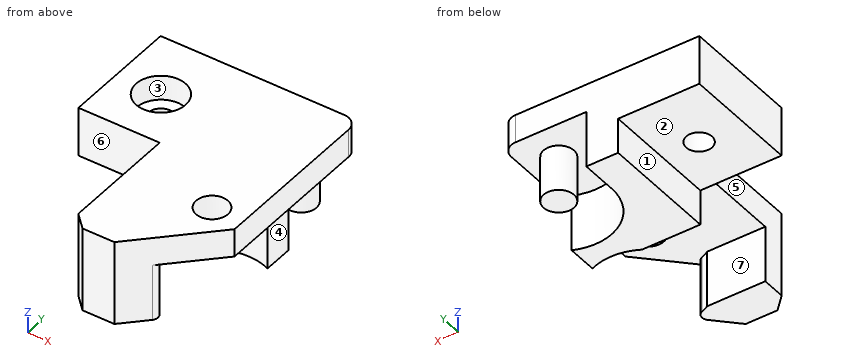
```python
from build123d import *

# Parameters (mm, degrees)
BOSS_EXTRUDE1_DEPTH                            = 4
SKETCH2_R                                      = 2.25
CUT_EXTRUDE1_DEPTH                             = 46
SKETCH2_3_R                                    = 2.15
BOSS_EXTRUDE2_DEPTH                            = 8
BOSS_EXTRUDE4_DEPTH                            = 8
SKETCH6_W                                      = 11.5
SKETCH6_H                                      = 18.413961031
CUT_EXTRUDE2_DEPTH                             = 47.400431032
SKETCH12_W                                     = 8
SKETCH12_H                                     = 13.1
CUT_EXTRUDE3_DEPTH                             = 40.286161686
CBORE_FOR_6_SOCKET_HEAD_CAP_SCREW1_D           = 3.6576
CBORE_FOR_6_SOCKET_HEAD_CAP_SCREW1_CBORE_D     = 7
CBORE_FOR_6_SOCKET_HEAD_CAP_SCREW1_CBORE_DEPTH = 3.5052
SKETCH13_W                                     = 11.5
SKETCH13_H                                     = 16.586038969
CUT_EXTRUDE4_DEPTH                             = 5
CHAMFER1_SIZE                                  = 2
CUT_EXTRUDE5_START                             = -1.5
SKETCH14_R                                     = 2.15
CUT_EXTRUDE5_DEPTH                             = 1.5


with BuildPart() as part:
    # Sketch1 → Boss-Extrude1 (new body)
    with BuildSketch(Plane.XY):
        with BuildLine():
            Line((18, 0), (28, 10))
            Line((28, 10), (28, 33))
            ThreePointArc((28, 33), (27.414213562, 34.414213562), (26, 35))
            Line((26, 35), (0, 35))
            Line((0, 35), (0, 0))
            Line((0, 0), (18, 0))
        make_face()
    extrude(amount=BOSS_EXTRUDE1_DEPTH)

    # Sketch2 → Cut-Extrude1 (cut, through all)
    with BuildSketch(Plane(origin=(0, 0, 0), x_dir=(-1, 0, 0), z_dir=(0, 0, -1))):
        with Locations((-23.5, 11.863961031)):
            Circle(SKETCH2_R)
    extrude(amount=-CUT_EXTRUDE1_DEPTH, mode=Mode.SUBTRACT)

    # Sketch2<3> → Boss-Extrude2 (add)
    with BuildSketch(Plane(origin=(0, 0, 0), x_dir=(-1, 0, 0), z_dir=(0, 0, -1))):
        with Locations(Location((-23.5, 29.863961031, 0), (0, 0, 180))):
            Circle(SKETCH2_3_R)
    extrude(amount=BOSS_EXTRUDE2_DEPTH)

    # Sketch2<5> → Boss-Extrude4 (add)
    with BuildSketch(Plane(origin=(0, 0, 0), x_dir=(-1, 0, 0), z_dir=(0, 0, -1))):
        with BuildLine():
            ThreePointArc((-26.5, 18.792344681), (-23.077745882, 19.402143932), (-19.745003329, 18.413961031))
            Line((-19.745003329, 18.413961031), (-15.95, 18.413961031))
            Line((-15.95, 18.413961031), (-15.95, 5.313961031))
            Line((-15.95, 5.313961031), (-19.725, 5.313961031))
            ThreePointArc((-19.725, 5.313961031), (-20.25595921, 5.035394245), (-20.807324798, 4.799782009))
            ThreePointArc((-20.807324798, 4.799782009), (-21.429052247, 4.074422526), (-21.15825613, 3.15825613))
            Line((-21.15825613, 3.15825613), (-18, 0))
            Line((-18, 0), (0, 0))
            Line((0, 0), (0, 35))
            Line((0, 35), (-16, 35))
            Line((-16, 35), (-16, 29.863961031))
            ThreePointArc((-16, 29.863961031), (-19.392080819, 23.589010832), (-26.5, 22.990097488))
            Line((-26.5, 22.990097488), (-26.5, 18.792344681))
        make_face()
    extrude(amount=BOSS_EXTRUDE4_DEPTH)

    # Sketch6 → Cut-Extrude2 (cut, through all)
    with BuildSketch(Plane(origin=(0, 0, -8), x_dir=(-1, 0, 0), z_dir=(0, 0, -1))):
        with Locations((-5.75, 9.206980515)):
            Rectangle(SKETCH6_W, SKETCH6_H)
    extrude(amount=-CUT_EXTRUDE2_DEPTH, mode=Mode.SUBTRACT)

    # Sketch12 → Cut-Extrude3 (cut, through all)
    with BuildSketch(Plane(origin=(15.95, 0, 0), x_dir=(0, 0, -1), z_dir=(1, 0, 0))):
        with Locations((4, 11.863961031)):
            Rectangle(SKETCH12_W, SKETCH12_H)
    extrude(amount=-CUT_EXTRUDE3_DEPTH, mode=Mode.SUBTRACT)

    # CBORE for #6 Socket Head Cap Screw1 (through all)
    with Locations(Plane.XY.offset(4)):
        with Locations((6.35, 26)):
            CounterBoreHole(CBORE_FOR_6_SOCKET_HEAD_CAP_SCREW1_D / 2, CBORE_FOR_6_SOCKET_HEAD_CAP_SCREW1_CBORE_D / 2, CBORE_FOR_6_SOCKET_HEAD_CAP_SCREW1_CBORE_DEPTH)

    # Sketch13 → Cut-Extrude4 (cut)
    with BuildSketch(Plane(origin=(0, 0, -8), x_dir=(-1, 0, 0), z_dir=(0, 0, -1))):
        with Locations((-5.75, 26.706980515)):
            Rectangle(SKETCH13_W, SKETCH13_H)
    extrude(amount=-CUT_EXTRUDE4_DEPTH, mode=Mode.SUBTRACT)

    # Chamfer1
    chamfer1_edges = [part.edges().sort_by_distance(p)[0] for p in [
        (11.5, 0, -2),
    ]]
    chamfer(chamfer1_edges, length=CHAMFER1_SIZE)

    # Sketch14 → Cut-Extrude5 (cut)
    with BuildSketch(Plane(origin=(0, 0, -8), x_dir=(-1, 0, 0), z_dir=(0, 0, -1)).offset(CUT_EXTRUDE5_START)):
        with Locations(Location((-23.5, 29.863961031, 0), (0, 0, 180))):
            Circle(SKETCH14_R)
    extrude(amount=CUT_EXTRUDE5_DEPTH, mode=Mode.SUBTRACT)


solid = part.part
```
Check sheet for the modelled part. Datum: model origin and axes. Units: mm. Face numbers are marked on the shaded views. A direction names the side the tool comes from. Round coordinates to 2 decimals unless told otherwise and drop trailing zeros. Order: outer loops, then holes, each group sorted by start corner. A loop starts at its lowest first (then second) coordinate and runs counter-clockwise, first axis right, second up. Notation, with made-up numbers: (44, 20.25) - (86, 20.25) arc R21 cw to (86, 30.25) - close; hole circle Ø10 at (9, -22). An arc over 180 degrees is marked (long way). Answer as CSV lines item,"result". Start each with the question number.
1) Scan lines: probe 1 along Y at (x, z) = (6.35, 2.05); probe 2 along Y at (x, z) = (6.35, -1.8); probe 3 along Z at (x, y) = (8, 24). Record each from-to range of solid material in increasing order.
2) Section check B-B (z = -1). Record the cut outline in (x, y) (3 decimals), then the cut area to 3 significant figures.
3) Tool access check on the marked faces 4, 5, 6 and 7. Record the directions out of +Z, -Z, +X, -X, +Y, -Y that give a thin tool (end or side, any length) a straight path to the whole face; none if there is none.
4) Draft check along X on the marked faces 1, 2 and 3. Enter one of: +X half, -X half, draft (parallel to the pull), parting line (faces both ways), or undercut.
5) Section check A-A (x = 6.35). Record the cut outline in (y, z).
6) Section check D-D (z = 1.25). Record the cut outline in (x, y).
7) Section check C-C (y = 26). Record the cut outline in (x, z).
8) Depth check by flat-ended pin: pin 1 (12 mm diameter, centred on x = 23.5, y = 13.5, fed in from -Z); pin 2 (2.5 mm diameter, centred on y = 30, z = -6.5, fed in from -X); pin 3 (6 mm diameter, centred on x = 7, z = -5, fed in from -Y); pin 4 (3.5 mm diameter, centred on x = 24, y = 29.5, fed in from -Z). Enter the tip coordinate at first touch or a pass-through.
Determined:
1,probe 1,"18.41 to 22.5, 29.5 to 35"
1,probe 2,"18.41 to 24.17, 27.83 to 35"
1,probe 3,"-3 to 0.49"
2,outline,"(0, 18.414) - (19.745, 18.414) arc R7.55 cw to (26.5, 18.792) - (26.5, 22.99) arc R7.5 cw to (16, 29.864) - (16, 35) - (0, 35) - close; (11.5, 2) - (13.5, 0) - (18, 0) - (21.158, 3.158) arc R1 ccw to (20.807, 4.8) arc R7.56 cw to (19.725, 5.314) - (11.5, 5.314) - close; circle Ø4.3 at (23.5, 29.864); hole circle Ø3.658 at (6.35, 26)"
2,area,"363 mm^2"
3,face 4,"-Z, +X, +Y, -Y"
3,face 5,"+Z, -Z, -X, -Y"
3,face 6,"-Z, -X"
3,face 7,"-Z, +X, -X"
4,face 1,"-X half"
4,face 2,"draft"
4,face 3,"undercut"
5,outline,"(18.41, -3) - (24.17, -3) - (24.17, 0.49) - (22.5, 0.49) - (22.5, 4) - (18.41, 4) - close; (27.83, -3) - (35, -3) - (35, 4) - (29.5, 4) - (29.5, 0.49) - (27.83, 0.49) - close"
6,outline,"(0, 18.41) - (11.5, 18.41) - (11.5, 2) - (13.5, 0) - (18, 0) - (28, 10) - (28, 33) arc R2 ccw to (26, 35) - (0, 35) - close; hole circle Ø7 at (6.35, 26); hole circle Ø4.5 at (23.5, 11.86)"
7,outline,"(0, -3) - (4.52, -3) - (4.52, 0.49) - (2.85, 0.49) - (2.85, 4) - (0, 4) - close; (8.18, -3) - (11.5, -3) - (11.5, -8) - (17.07, -8) - (17.07, 0) - (28, 0) - (28, 4) - (9.85, 4) - (9.85, 0.49) - (8.18, 0.49) - close"
8,pin 1,"z = -8"
8,pin 2,"x = 11.5"
8,pin 3,"y = 18.41"
8,pin 4,"z = -6.5"
